Here's how the part is built. I have some questions about the finished solid (model axes, mm). A direction names the side the tool comes from. Give positions to 0.01 mm unless a question says otherwise; leave off trailing zeros.
Autodesk Inventor part; units mm, degrees
ref_plane "YZ Plane" through (0, 0, 0) normal (1, 0, 0) x (0, 1, 0)
ref_plane "XZ Plane" through (0, 0, 0) normal (0, 1, 0) x (-1, 0, 0)
ref_plane "XY Plane" through (0, 0, 0) normal (0, 0, 1) x (1, 0, 0)
sketch "Sketch1" plane through (0, 0, 0) normal (0, 1, 0) x (-1, 0, 0)
  line L0 (170, 250) -> (-170, 250)
  line L1 (-170, 250) -> (-170, -250)
  line L2 (-170, -250) -> (170, -250)
  line L3 (170, -250) -> (170, 250)
  line L4 (170, 250) -> (-170, -250) construction
  line L5 (-170, 250) -> (170, -250) construction
  point P0 (0, 0)
  dimension "d0" = 340
  dimension "d1" = 500
extrude "Extrusion1" add sketch "Sketch1" along normal blind 11.1125
sketch "Sketch2" plane through (0, 11.1125, 0) normal (0, 1, 0) x (1, 0, 0)
  line L0 (-170, -250) -> (170, -250)
  line L1 (170, -250) -> (170, 250)
  line L2 (170, 250) -> (-170, 250)
  line L3 (-170, 250) -> (-170, -250)
  point P0 (0, 0)
  point P1 (-160, -240)
  dimension "d4" = 10
  dimension "d5" = 10
hole "Hole1" at (-160, 11.1125, 240) direction (0, -1, 0) diameter 5.5 end through all counterbore diameter 10 counterbore depth 5
pattern_linear "Rectangular Pattern1" count 2 spacing 480 along (0, 0, -1) count 5 spacing 80 along (1, 0, 0) of "Hole1"
sketch "Sketch3" plane through (-170, 0, -250) normal (-1, 0, 0) x (0, 0, 1)
  line L0 (0, 0) -> (500, 0)
  line L1 (500, 0) -> (500, 11.1125)
  line L2 (0, 11.1125) -> (500, 11.1125)
  line L3 (0, 0) -> (0, 11.1125)
  line L4 (0, 0) -> (0, 11.1125)
  arc A0 (0, 3.175) -> (0, 6.35) centre (0, 4.7625) ccw
  point P0 (250, 0)
  dimension "d19" = 1.5875
  dimension "d20" = 6.35
extrude "oRingGroove" cut sketch "Sketch3" against normal through all contours L3 A0
mirror "Mirror1" about plane through (0, 0, 0) normal (0, 0, 1) of "oRingGroove"
equation "\"d1\" = depth"
equation "\"d2\" = facingThickness - facingGasketThickness"
equation "\"d19\" = 0.125 * facingThickness"
equation "\"d20\" = 0.5 * facingThickness"
equation "\"depth\" = 500"
equation "\"facingThickness\" = 12.7"
equation "\"facingGasketThickness\" = 1.5875"
properties part number "sideFace" material "Wood (Cherry)"
Q1. I'm going to push flat-ended pins straight in: P1, Ø7, axis at x = 160, z = -240, coming from the +Y side; P2, Ø4.5, axis at x = 160, z = 240, coming from the +Y side; P3, Ø1, axis at x = 111.5, y = 4.5, coming from the -Z side. Where does each tip first touch, or does it pass through?
Filled sheet:
P1: stops at y = 6.11
P2: passes through
P3: stops at z = -248.61
Q2. For faces 4 (the face through (2, 0, 4)), 5 (the face through (162.2, 6.112, 242.2)), which set-ups out of +Z, -Z, +X, -X, +Y, -Y let a thin tool reach every point of the face, with its end or its side?
Filled sheet:
face 4: +Z, -Z, +X, -X, -Y
face 5: +Y
Q3. Thinking about a two-plate mould opening in X: for faces 1 (the face through (170, 5, 3)), 2 (the face through (2.2, 6.112, -237.8)), 3 (the face through (2, 11.112, 4)), which applies, released by +X, released by -X, zero draft, split by the parting line, or undercut?
Filled sheet:
face 1: released by +X
face 2: undercut
face 3: zero draft
Q4. I need wall thicknesses on L1, parallel to Z at x = -80, y = 7.65; L2, parallel to X at y = 10.1, z = 240; L3, parallel to Z at x = -52, y = 4.25. Which ranges of each line are inside material? Lowest first, please.
Filled sheet:
L1: z = -250 to -245, -235 to 235, 245 to 250
L2: x = -170 to -165, -155 to -85, -75 to -5, 5 to 75, 85 to 155, 165 to 170
L3: z = -248.5 to 248.5
